Autodesk Inventor part; units mm, degrees
ref_plane "YZ Plane" through (0, 0, 0) normal (1, 0, 0) x (0, 1, 0)
ref_plane "XZ Plane" through (0, 0, 0) normal (0, 1, 0) x (-1, 0, 0)
ref_plane "XY Plane" through (0, 0, 0) normal (0, 0, 1) x (1, 0, 0)
sketch "Skizze1" plane through (0, 0, 0) normal (0, 1, 0) x (-1, 0, 0)
  line L0 (0, 0) -> (2, 0)
  line L1 (2, 0) -> (2, -1)
  line L2 (2, -1) -> (1.6, -1)
  line L3 (1.6, -1) -> (1.6, -1.65)
  line L4 (1.6, -1.65) -> (2, -1.65)
  line L5 (2, -1.65) -> (2, -26.65)
  line L6 (2, -26.65) -> (1.6, -26.65)
  line L7 (1.6, -26.65) -> (1.6, -27.3)
  line L8 (1.6, -27.3) -> (2, -27.3)
  line L9 (2, -27.3) -> (2, -28.3)
  line L10 (2, -28.3) -> (0, -28.3)
  line L11 (0, 0) -> (0, -28.3)
  dimension "d0" = 2
  dimension "d1" = 1
  dimension "d2" = 0.65
  dimension "d3" = 0.65
  dimension "d5" = 1
  dimension "d6" = 4
  dimension "d7" = 3.2
  dimension "d9" = 25
revolve "Umdrehung1" add sketch "Skizze1" angle 360 about axis through (0, 0, 0) along (0, 0, -1)
properties part number "Kipphebelachse"
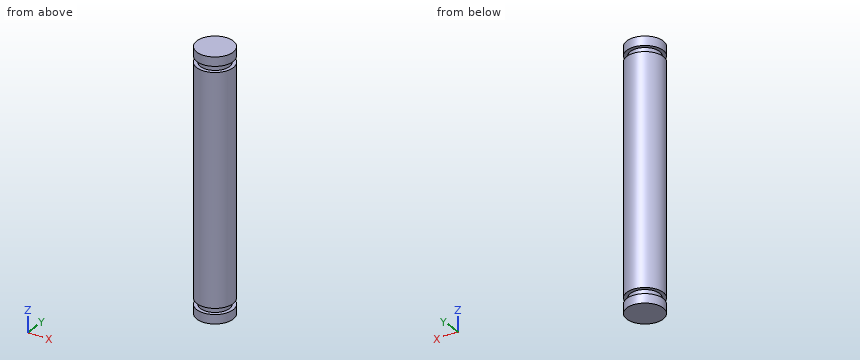
Can you work these out from the model? Positions are in its coordinate system, mm. Give positions to 0.01 mm unless a question says otherwise; leave off trailing zeros. Loops run counter-clockwise (first coordinate to the right, second up) from the corner with the lowest first, then second, coordinate; pieces in that order, holes last. Notation, with made-up numbers: M 20,-31 L 33,-31 A15 ccw 33,-26 Z; hole C 70.25,33 d5. An arc over 180 degrees is marked long. Answer in a Markdown table with one row per item.
1. If I drill on line 1 along Z through (x, y) = (-0.3, -1.7); line 2 along Y through (x, z) = (0.15, -6.25); line 3 along X through (y, z) = (-0.05, -27), over which ranges is the centre line in solid material (lowest first)?
Taken from the geometry:
| item | result |
|---|---|
| line 1 | z = -28.3 to -27.3, -26.65 to -1.65, -1 to 0 |
| line 2 | y = -1.99 to 1.99 |
| line 3 | x = -1.6 to 1.6 |
2. Suppose I cut it at B-B on y = -1.2. Write out the boundary of the cut face in (x, z), plus the area to 3 significant figures.
Taken from the geometry:
| item | result |
|---|---|
| outline | M -1.6,-28.3 L 1.6,-28.3 L 1.6,-27.3 L 1.06,-27.3 L 1.06,-26.65 L 1.6,-26.65 L 1.6,-1.65 L 1.06,-1.65 L 1.06,-1 L 1.6,-1 L 1.6,0 L -1.6,0 L -1.6,-1 L -1.06,-1 L -1.06,-1.65 L -1.6,-1.65 L -1.6,-26.65 L -1.06,-26.65 L -1.06,-27.3 L -1.6,-27.3 Z |
| area | 89.2 mm² |
3. Suppose I cut it at A-A on x = 1.1. Write out the boundary of the cut face in (y, z), plus the area to 3 significant figures.
Taken from the geometry:
| item | result |
|---|---|
| outline | M -1.67,-28.3 L 1.67,-28.3 L 1.67,-27.3 L 1.16,-27.3 L 1.16,-26.65 L 1.67,-26.65 L 1.67,-1.65 L 1.16,-1.65 L 1.16,-1 L 1.67,-1 L 1.67,0 L -1.67,0 L -1.67,-1 L -1.16,-1 L -1.16,-1.65 L -1.67,-1.65 L -1.67,-26.65 L -1.16,-26.65 L -1.16,-27.3 L -1.67,-27.3 Z |
| area | 93.2 mm² |
